from build123d import *

# Parameters (mm, degrees)
F4_W     = 117.5877898932
F4_H     = 62.227293849
F0_DEPTH = 63.5
F5_W     = 92.6998779178
F5_H     = 39.9431586266
F1_DEPTH = 63.501
F2_R     = 7.7272697415
F3_DEPTH = 117.5887898932
F6_W     = 50.2068921924
F6_H     = 22.9567790627
F7_DEPTH = 62.228293849


with BuildPart() as f0:
    # F4 (on Top) → F0 (new body)
    with BuildSketch(Plane.XY):
        with Locations((1.7765834928, -0.2040341496)):
            Rectangle(F4_W, F4_H)
    extrude(amount=F0_DEPTH)

    # F5 (on face) → F1 (cut, through all)
    with BuildSketch(Plane.XY.offset(63.5)):
        with Locations((2.2740103304, -0.2917349339)):
            Rectangle(F5_W, F5_H)
    extrude(amount=-F1_DEPTH, mode=Mode.SUBTRACT)

    # F2 (on face) → F3 (cut, through all)
    with BuildSketch(Plane.YZ.offset(60.5704784393)):
        with Locations((0, 33.4859117866)):
            Circle(F2_R)
    extrude(amount=-F3_DEPTH, mode=Mode.SUBTRACT)

    # F6 (on face) → F7 (cut, through all)
    with BuildSketch(Plane.XZ.offset(31.3176810741)):
        with Locations((1.0511763394, 52.0216104686)):
            Rectangle(F6_W, F6_H)
    extrude(amount=-F7_DEPTH, mode=Mode.SUBTRACT)


solid = f0.part
Build history of the part. All positions in model axes, mm. A direction names the side the tool comes from. Give positions to 0.01 mm unless a question says otherwise; leave off trailing zeros. Loops run counter-clockwise (first coordinate to the right, second up) from the corner with the lowest first, then second, coordinate; pieces in that order, holes last. Notation, with made-up numbers: (26, 53) - (53, 53) arc R21 ccw to (53, 60) - close; hole circle Ø1 at (52, 68). An arc over 180 degrees is marked (long way). Write item = value, one per line. Start each with the question number.
1) Pull direction Y, two halves, no side cores. Call faces 1 (the cylindrical face through (54.681, -1.675, 25.942)), 2 (the flat face through (-44.076, -1, 25)), 3 (the flat face through (1, 30.91, 31)), 4 (the flat face through (1, -26, 40.543)): +Y half, -Y half, draft (parallel to the pull), parting line (faces both ways), or undercut.
2) Band-saw the part on A-A on y = 12.5. Give the cut face in (x, z).
3) Band-saw the part on C-C on z = 43. Give the cut face in (x, y), plus the area to 3 significant figures.
4) Band-saw the part on B-B on x = -30. Give the cut face in (y, z).
5) Drop flat-ended pins along their axis: pin 1 Ø5.5 at (x, y) = (-8.5, 27) entering from +Z; pin 2 Ø20 at (y, z) = (0, 33.49) entering from +X. Give the stop position or say it passes through.
6) Tool access for faces 5 (the flat face through (48.624, -1, 25)), 6 (the flat face through (1, 21, 0)), 7 (the flat face through (26.155, -26, 52)): list every direction of +Z, -Z, +X, -X, +Y, -Y with a clear straight run to the whole face (end or side of a thin tool).
7) Band-saw the part on D-D on y = 0. Give the cut face in (x, z).
8) Probe probe 1 along Y at (x, z) = (-24.5, 12); probe 2 along X at (y, z) = (19.5, 52); probe 3 along Z at (x, y) = (-54, 0). List the from-to ranges inside material, lowest first. Write a range as from..to.
Final values:
q1.face_1 = undercut
q1.face_2 = undercut
q1.face_3 = +Y half
q1.face_4 = draft
q2.outline = (-57.02, 0) - (-44.08, 0) - (-44.08, 63.5) - (-57.02, 63.5) - close; (48.62, 0) - (60.57, 0) - (60.57, 63.5) - (48.62, 63.5) - close
q3.outline = (-57.02, -31.32) - (-24.05, -31.32) - (-24.05, -20.26) - (-44.08, -20.26) - (-44.08, 19.68) - (-24.05, 19.68) - (-24.05, 30.91) - (-57.02, 30.91) - close; (26.15, -31.32) - (60.57, -31.32) - (60.57, 30.91) - (26.15, 30.91) - (26.15, 19.68) - (48.62, 19.68) - (48.62, -20.26) - (26.15, -20.26) - close
q3.area = 2,500 mm²
q4.outline = (-31.32, 0) - (-20.26, 0) - (-20.26, 63.5) - (-31.32, 63.5) - close; (19.68, 0) - (30.91, 0) - (30.91, 63.5) - (19.68, 63.5) - close
q5.pin_1 = 40.54
q5.pin_2 = 60.57
q6.face_5 = +Z, -Z
q6.face_6 = -Z, +X, -X, +Y, -Y
q6.face_7 = +Z, +Y, -Y
q7.outline = (-57.02, 0) - (-44.08, 0) - (-44.08, 25.76) - (-57.02, 25.76) - close; (-57.02, 41.21) - (-44.08, 41.21) - (-44.08, 63.5) - (-57.02, 63.5) - close; (48.62, 0) - (60.57, 0) - (60.57, 25.76) - (48.62, 25.76) - close; (48.62, 41.21) - (60.57, 41.21) - (60.57, 63.5) - (48.62, 63.5) - close
q8.probe_1 = -31.32..-20.26, 19.68..30.91
q8.probe_2 = -57.02..-44.08, 48.62..60.57
q8.probe_3 = 0..25.76, 41.21..63.5
